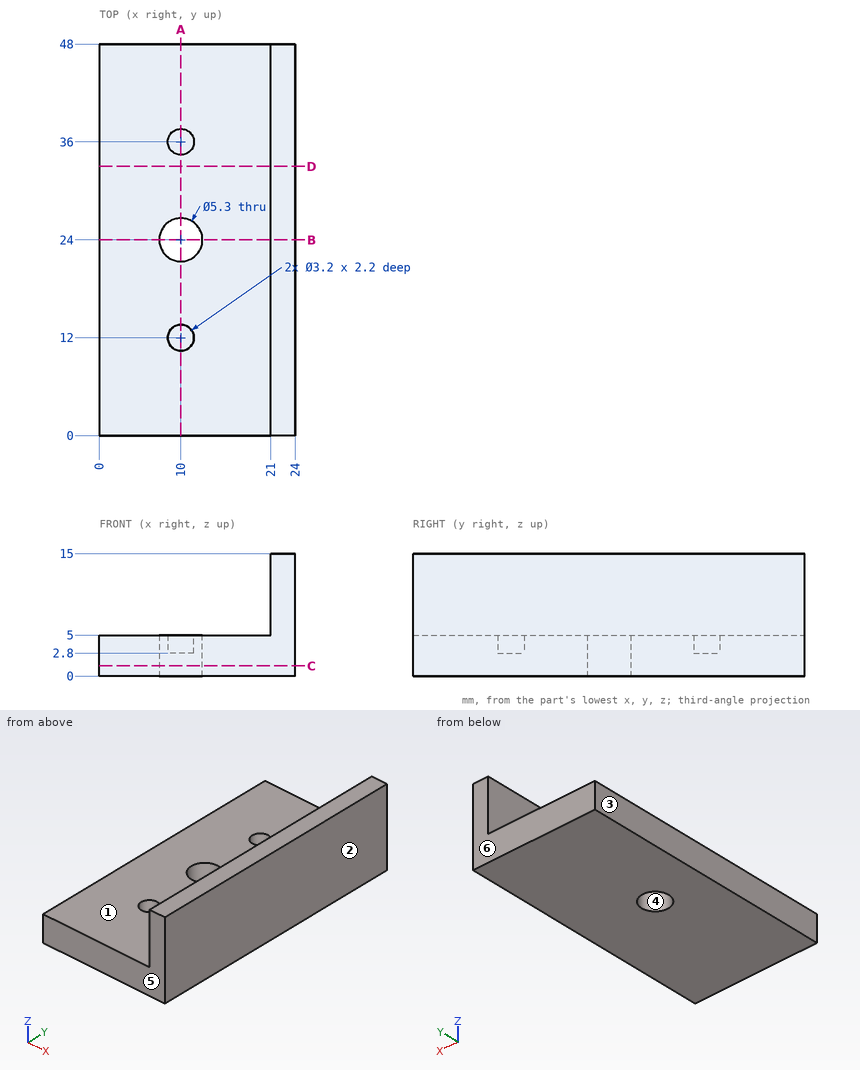
Print and shaded views of the part. All mm, measured from the part's lowest x, y and z. A direction names the side the tool comes from. Coordinates: 2 decimals unless noted, no trailing zeros. Order: outer loops, then holes, each group sorted by start corner. A loop starts at its lowest first (then second) coordinate and runs counter-clockwise, first axis right, second up. Notation, with made-up numbers: (38, -11) -> (65, -11) arc R26 ccw to (65, 5) -> close; hole circle Ø6 at (-38.5, 25). An arc over 180 degrees is marked (long way). Answer as a JSON object with one key per item and string values. Group by question number.
1) Cut at D-D, the plane y = 33. Write the cut outline in (x, z).
2) Drill centre lines: L1, parallel to Y at x = 10, z = 4.55; L2, parallel to X at y = 12, z = 3.8; L3, parallel to X at y = 17, z = 9.75. Where is each one in solid material? Low to high.
3) Which spindle directions (+Z, -Z, +X, -X, +Y, -Y) get a long thin tool onto all of the face, cutting with end or side? Do the marked faces 1 and 2. Say none if no direction does.
4) Flat gauge pins, fed straight in: pin 1 (8 mm diameter, centred on y = 11, z = 11, fed in from -X); pin 2 (6 mm diameter, centred on y = 9, z = 6.5, fed in from -X); pin 3 (5 mm diameter, centred on x = 10, y = 24, fed in from +Z); pin 4 (1 mm diameter, centred on x = 10.5, y = 36.5, fed in from +Z). Where does each tip first touch, or does it go through?
5) Pull direction Y, two halves, no side cores. Call the marked faces 3, 4, 5 and 6: +Y half, -Y half, draft (parallel to the pull), parting line (faces both ways), or undercut.
6) Cut at C-C, the plane z = 1.25. Write the cut outline in (x, y).
7) Cut at B-B, the plane y = 24. Write the cut outline in (x, z).
8) Cut at A-A, the plane x = 10. Write the cut outline in (y, z).
Check values:
{
 "1": {"outline": "(0, 0) -> (24, 0) -> (24, 15) -> (21, 15) -> (21, 5) -> (0, 5) -> close"},
 "2": {"L1": "y = 0 to 10.4, 13.6 to 21.35, 26.65 to 34.4, 37.6 to 48", "L2": "x = 0 to 8.4, 11.6 to 24", "L3": "x = 21 to 24"},
 "3": {"face 1": "+Z, -X, +Y, -Y", "face 2": "+Z, -Z, +X, +Y, -Y"},
 "4": {"pin 1": "stops at x = 21", "pin 2": "stops at x = 0", "pin 3": "passes through", "pin 4": "stops at z = 2.8"},
 "5": {"face 3": "draft", "face 4": "undercut", "face 5": "-Y half", "face 6": "+Y half"},
 "6": {"outline": "(0, 0) -> (24, 0) -> (24, 48) -> (0, 48) -> close; hole circle Ø5.3 at (10, 24)"},
 "7": {"outline": "(0, 0) -> (7.35, 0) -> (7.35, 5) -> (0, 5) -> close; (12.65, 0) -> (24, 0) -> (24, 15) -> (21, 15) -> (21, 5) -> (12.65, 5) -> close"},
 "8": {"outline": "(0, 0) -> (21.35, 0) -> (21.35, 5) -> (13.6, 5) -> (13.6, 2.8) -> (10.4, 2.8) -> (10.4, 5) -> (0, 5) -> close; (26.65, 0) -> (48, 0) -> (48, 5) -> (37.6, 5) -> (37.6, 2.8) -> (34.4, 2.8) -> (34.4, 5) -> (26.65, 5) -> close"}
}
